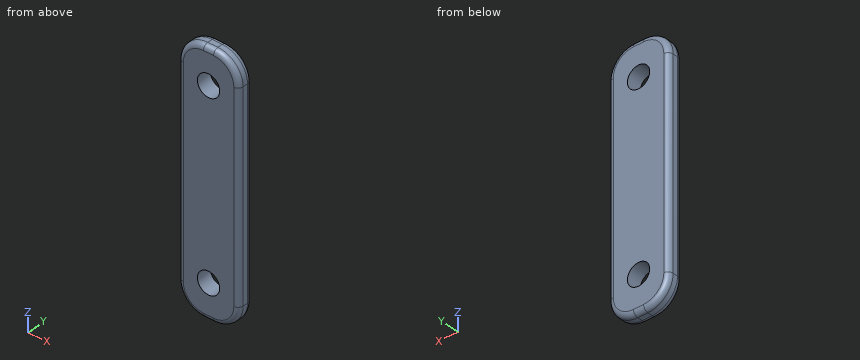
from build123d import *

# Parameters (mm, degrees)
F0_W           = 12
F0_H           = 50.5
F1_DEPTH       = 3
F4_D           = 4.4
F4_DEPTH       = 70
F4_CBORE_D     = 8.25
F4_CBORE_DEPTH = 4
F5_R           = 5
F6_R           = 1


with BuildPart() as f1:
    # F0 (on Front) → F1 (new body)
    with BuildSketch(Plane.XZ):
        Rectangle(F0_W, F0_H)
    extrude(amount=F1_DEPTH)

    # F4
    with Locations(Plane(origin=(0, 8, 0), x_dir=(1, 0, 0), z_dir=(0, 1, 0))):
        with Locations((0, 18.228), (0, -18.228)):
            CounterBoreHole(F4_D / 2, F4_CBORE_D / 2, F4_CBORE_DEPTH, depth=F4_DEPTH)

    # F5
    f5_edges = [f1.edges().sort_by_distance(p)[0] for p in [
        (-6, -1.5, 25.25),
        (6, -1.5, 25.25),
        (-6, -1.5, -25.25),
        (6, -1.5, -25.25),
    ]]
    fillet(f5_edges, radius=F5_R)

    # F6
    f6_edges = [f1.edges().sort_by_distance(p)[0] for p in [
        (6, 0, 0),
        (6, -3, 0),
    ]]
    fillet(f6_edges, radius=F6_R)


solid = f1.part
Can you work these out from the model? Positions are in its coordinate system, mm. Coordinates: 2 decimals unless noted, no trailing zeros. Write each loop counter-clockwise with the first axis right and the second up, starting at its lowest first coordinate (ties: lowest second). Pieces come first, ordered by that corner, then holes. Notation, with made-up numbers: (10, 60) - (15, 60) arc R16 cw to (15, 81) - close; hole circle Ø5 at (-30, 40). An arc over 180 degrees is marked (long way). Return JSON: item names as keys, results as strings. Group by question number.
Item 1: Please list where these lines run through material, in increasing order: probe 1 along Z at (x, y) = (0, -2); probe 2 along Z at (x, y) = (-1, -0.75); probe 3 along Z at (x, y) = (-4, -1.2).
Item 2: If we section it at B-B (z = -3): Write out the boundary of the cut face in (x, y).
Item 3: If we section it at A-A (x = 0): Write out the boundary of the cut face in (y, z), then the cut area to 3 significant figures.
Return value:
{
 "1": {"probe 1": "z = -25.25 to -20.43, -16.03 to 16.03, 20.43 to 25.25", "probe 2": "z = -25.22 to -20.19, -16.27 to 16.27, 20.19 to 25.22", "probe 3": "z = -24.25 to 24.25"},
 "2": {"outline": "(-6, -2) arc R1 ccw to (-5, -3) - (5, -3) arc R1 ccw to (6, -2) - (6, -1) arc R1 ccw to (5, 0) - (-5, 0) arc R1 ccw to (-6, -1) - close"},
 "3": {"outline": "(-3, -24.25) arc R1 ccw to (-2, -25.25) - (-1, -25.25) arc R1 ccw to (0, -24.25) - (0, -20.43) - (-3, -20.43) - close; (-3, -16.03) - (0, -16.03) - (0, 16.03) - (-3, 16.03) - close; (-3, 20.43) - (0, 20.43) - (0, 24.25) arc R1 ccw to (-1, 25.25) - (-2, 25.25) arc R1 ccw to (-3, 24.25) - close", "area": "124 mm^2"}
}
